Could you check a few things on this drawing? It's one solid part, dimensions in mm from its lowest x, y, z. A direction names the side the tool comes from. Round coordinates to 2 decimals unless told otherwise and drop trailing zeros. Write each loop counter-clockwise with the first axis right and the second up, starting at its lowest first coordinate (ties: lowest second). Pieces come first, ordered by that corner, then holes. Notation, with made-up numbers: (48, 4.5) -> (79, 4.5) arc R10 ccw to (79, 10.5) -> close; hole circle Ø1 at (62.25, 31). An arc over 180 degrees is marked (long way). Answer in a Markdown table with one row per item.
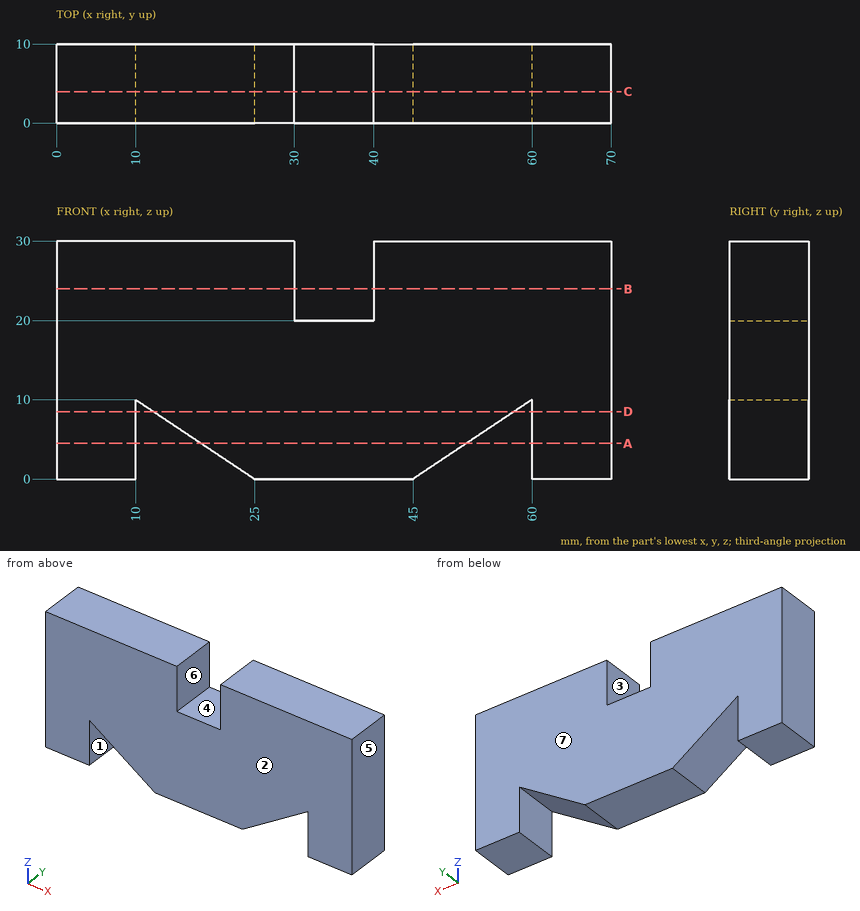
1) I want a section at A-A, the plane z = 4.5. List the corners of the cut face in (x, y) for me.
Response:
| item | result |
|---|---|
| outline | (0, 0) -> (10, 0) -> (10, 10) -> (0, 10) -> close; (18.25, 0) -> (51.75, 0) -> (51.75, 10) -> (18.25, 10) -> close; (60, 0) -> (70, 0) -> (70, 10) -> (60, 10) -> close |
2) I want a section at D-D, the plane z = 8.5. List the corners of the cut face in (x, y) for me.
Response:
| item | result |
|---|---|
| outline | (0, 0) -> (10, 0) -> (10, 10) -> (0, 10) -> close; (12.25, 0) -> (57.75, 0) -> (57.75, 10) -> (12.25, 10) -> close; (60, 0) -> (70, 0) -> (70, 10) -> (60, 10) -> close |
3) We'd pull the mould along X, two halves only. Please class the marked faces 4, 5, 6 and 7: +X half, -X half, draft (parallel to the pull), parting line (faces both ways), or undercut.
Response:
| item | result |
|---|---|
| face 4 | undercut |
| face 5 | +X half |
| face 6 | undercut |
| face 7 | draft |
4) I want a section at C-C, the plane y = 4. List the corners of the cut face in (x, z) for me, and give its area (3 significant figures).
Response:
| item | result |
|---|---|
| outline | (0, 0) -> (10, 0) -> (10, 10) -> (25, 0) -> (45, 0) -> (60, 10) -> (60, 0) -> (70, 0) -> (70, 30) -> (40, 30) -> (40, 20) -> (30, 20) -> (30, 30) -> (0, 30) -> close |
| area | 1,850 mm^2 |
5) I want a section at B-B, the plane z = 24. List the corners of the cut face in (x, y) for me, and give its area (3 significant figures).
Response:
| item | result |
|---|---|
| outline | (0, 0) -> (30, 0) -> (30, 10) -> (0, 10) -> close; (40, 0) -> (70, 0) -> (70, 10) -> (40, 10) -> close |
| area | 600 mm^2 |
6) Which directions (+Z, -Z, +X, -X, +Y, -Y) give clear straight access to the entire face, cutting with the end or side of a thin tool? Please do the marked faces 1, 2 and 3.
Response:
| item | result |
|---|---|
| face 1 | -Z, +Y, -Y |
| face 2 | +Z, -Z, +X, -X, -Y |
| face 3 | +Z, +Y, -Y |
7) I need wall thicknesses on line 1 (X direction, y = 7.25, z = 28.25); line 2 (X direction, y = 3, z = 4.25) (3 decimals); line 3 (X direction, y = 4, z = 8). Which ranges of each line are inside material? Lowest first, please. Write a range as [from, to].
Response:
| item | result |
|---|---|
| line 1 | x = [0, 30], [40, 70] |
| line 2 | x = [0, 10], [18.625, 51.375], [60, 70] |
| line 3 | x = [0, 10], [13, 57], [60, 70] |
8) For pin 1 (5 mm diameter, centred on x = 33, y = 3.5, fed in from +Z), with a flat end and sliding along its axis, tell me the tip position at first contact or that it passes through.
Response:
| item | result |
|---|---|
| pin 1 | stops at z = 20 |
